Can you work these out from the model? Positions are in its coordinate system, mm. Coordinates: 2 decimals unless noted, no trailing zeros. Loops run counter-clockwise (first coordinate to the right, second up) from the corner with the lowest first, then second, coordinate; pieces in that order, holes last. Notation, with made-up numbers: (-21, 74) -> (32, 74) arc R23 ccw to (32, 103) -> close; hole circle Ø6 at (-5, 41). An arc over 180 degrees is marked (long way). Put each result on its own line as item: value. Start each with the question number.
Item 1: If we section it at A-A on z = 0: Please give me the cut outline in (x, y).
Item 2: We'd pull the mould along Z, two halves only. Please class faces 1 (the flat face through (4.5, 5, 3)), 2 (the cylindrical face through (0.059, 6.466, -2.681)), 3 (the cylindrical face through (0.06, -1.08, -4.88)): pulls with the +Z half, pulls with the -Z half, needs draft (parallel to the pull), parting line crosses it, or undercut.
Item 3: If we section it at C-C on x = -1: Please give me the cut outline in (y, z).
Item 4: Will these pins go through, and if not, where does the flat tip stop? P1, Ø3, axis at y = 3, z = 1.5, coming from the +X side; P2, Ø1.5, axis at x = -3, z = 3.5, coming from the -Y side; P3, Ø2, axis at x = -2.5, y = 3.5, coming from the -Z side; P4, Ø3, axis at x = -3.5, z = -2.5, coming from the -Y side.
Item 5: Please list where these lines run through material, in increasing order: L1, parallel to Z at x = -1.25, y = 0; L2, parallel to Y at x = -4, z = -1.75; L3, parallel to Y at x = -2.5, z = 0.5. Write a range as from..to.
```python
from build123d import *

# Parameters (mm, degrees)
SKETCH_1_W     = 9
SKETCH_1_H     = 2
CHAMFER_1_SIZE = 0.3
FILLET_1_R     = 0.5


with BuildPart() as part:
    # 草圖1 → 旋轉1 (revolve)
    with BuildSketch(Plane.XY):
        with Locations((0, 6)):
            Rectangle(SKETCH_1_W, SKETCH_1_H)
    revolve(axis=Axis((-51.523727229, 0, 0), (1, 0, 0)))

    # 導角1
    chamfer_1_edges = [part.edges().sort_by_distance(p)[0] for p in [
        (4.5, -7, 0),
        (-4.5, -7, 0),
    ]]
    chamfer(chamfer_1_edges, length=CHAMFER_1_SIZE)

    # 圓角1
    fillet_1_edges = [part.edges().sort_by_distance(p)[0] for p in [
        (-4.5, -5, 0),
        (4.5, -5, 0),
    ]]
    fillet(fillet_1_edges, radius=FILLET_1_R)


solid = part.part
```
Solutions:
1. outline: (-4.5, -6.7) -> (-4.2, -7) -> (4.2, -7) -> (4.5, -6.7) -> (4.5, -5.5) arc R0.5 ccw to (4, -5) -> (-4, -5) arc R0.5 ccw to (-4.5, -5.5) -> close; (-4.5, 5.5) arc R0.5 ccw to (-4, 5) -> (4, 5) arc R0.5 ccw to (4.5, 5.5) -> (4.5, 6.7) -> (4.2, 7) -> (-4.2, 7) -> (-4.5, 6.7) -> close
2. face 1: needs draft
2. face 2: parting line crosses it
2. face 3: undercut
3. outline: circle Ø14 at (0, 0); hole circle Ø10 at (0, 0)
4. P1: through
4. P2: y = -6.44
4. P3: z = -6.54
4. P4: y = -6.93
5. L1: -7..-5, 5..7
5. L2: -6.78..-4.68, 4.68..6.78
5. L3: -6.98..-4.97, 4.97..6.98
